Work out the finished part from the listing and answer in its coordinate system (mm). A direction names the side the tool comes from. Coordinates: 2 decimals unless noted, no trailing zeros. Order: outer loops, then holes, each group sorted by start corner. A loop starts at its lowest first (then second) coordinate and runs counter-clockwise, first axis right, second up.
1. Find the intervals of material crossed by probe 1 along Y at (x, z) = (12, -4.75); probe 2 along Y at (x, z) = (9.25, -0.5); probe 3 along Z at (x, y) = (11, -12.75), in increasing order.
2. Flat-ended cylindrical pins translate along their axes: pin 1 Ø7 at (x, y) = (12, -8.5) entering from +Z; pin 2 Ø5 at (x, y) = (6.5, -2.5) entering from +Z; pin 3 Ø1.5 at (y, z) = (-7, -5.5) entering from -X; pin 4 Ø0.7 at (x, z) = (3, -1.5) entering from -Y. Find the tip coordinate at first contact, or state that the pin passes through.
3. The part is cut by section A-A, the plane x = 12.5. Give the vertices of the cut face in (y, z).
4. A tool of negligible diameter and unlimited length cuts with its end or side. For faces 1 (the flat face through (10, 0, -5)), 2 (the flat face through (1, -8, -3.175)), 3 (the flat face through (8, -1.778, -3)), 4 (the flat face through (9.398, -14, -1)), 5 (the flat face through (0, -8, -2)), from which of +Z, -Z, +X, -X, +Y, -Y can it reach the whole face along a straight path? Write none if from no direction.
5. The part is cut by section B-B, the plane y = -8.5. Give the vertices of the cut face in (x, z) (3 decimals), then the cut area to 3 significant figures.
6. The part is cut by section C-C, the plane z = -0.25. Give the vertices of the cut face in (x, y), then the cut area to 3 significant figures.
7. Determine the mould class of faces 6 (the flat face through (8, -13.462, -3)), 7 (the flat face through (10, -15, -2.794)), 8 (the flat face through (10, -1, -2.794)), 9 (the flat face through (4.125, -7.538, -3.091)) for opening direction Z: +Z half, -Z half, draft (parallel to the pull), parting line (faces both ways), or undercut.
```python
from build123d import *

# Parameters (mm, degrees)
BOSS_EXTRUDE1_DEPTH = 15.24
CUT_EXTRUDE1_DEPTH  = 16.748
CUT_EXTRUDE2_DEPTH  = 5.842
FILLET1_R           = 0.762


with BuildPart() as part:
    # Sketch1 → Boss-Extrude1 (new body)
    with BuildSketch(Plane(origin=(0, 0, 0), x_dir=(1, 0, 0), z_dir=(0, 1, 0))):
        Polygon((0, 0), (0, 3.175), (2.413, 3.175), (6.604, 7.366), (15.748, 7.366), (15.748, 2.794), (9.398, 2.794), (9.398, 0), align=None)
    extrude(amount=-BOSS_EXTRUDE1_DEPTH)

    # Sketch5 → Cut-Extrude1 (cut, through all)
    with BuildSketch(Plane.ZY):
        Polygon((0, -1.0033), (0, 0), (-2.794, 0), (-2.794, -1.0033), (-2.2606, -1.0033), (-1.7018, -0.4445), (-1.0922, -0.4445), (-0.5334, -1.0033), align=None)
    cut_extrude1 = extrude(amount=-CUT_EXTRUDE1_DEPTH, mode=Mode.SUBTRACT)

    # Mirror1: Cut-Extrude1 across plane
    add(cut_extrude1.mirror(Plane.ZX.offset(-7.62)), mode=Mode.SUBTRACT)

    # Sketch6 → Cut-Extrude2 (cut, symmetric)
    with BuildSketch(Plane(origin=(0, -7.62, 0), x_dir=(1, 0, 0), z_dir=(0, 1, 0))):
        Polygon((15.748, 6.096), (7.130051224, 6.096), (1.034051224, 0), (15.748, 0), align=None)
    extrude(amount=CUT_EXTRUDE2_DEPTH, both=True, mode=Mode.SUBTRACT)

    # Fillet1
    fillet1_edges = [part.edges().sort_by_distance(p)[0] for p in [
        (11.439025612, -13.462, -6.096),
        (11.439025612, -1.778, -6.096),
        (11.176, -15.24, -7.366),
        (11.176, 0, -7.366),
    ]]
    fillet(fillet1_edges, radius=FILLET1_R)


solid = part.part
```
Geometry says:
1. probe 1: y = -15.24 to -13.46, -1.78 to 0
1. probe 2: y = -14.24 to -13.46, -1.78 to -1
1. probe 3: z = -7.37 to -6.09
2. pin 1: stops at z = -6.1
2. pin 2: stops at z = 0
2. pin 3: stops at x = 3.99
2. pin 4: stops at y = -14.8
3. outline: (-15.24, -6.6) arc R0.76 ccw to (-14.48, -7.37) - (-0.76, -7.37) arc R0.76 ccw to (0, -6.6) - (0, -2.79) - (-1.78, -2.79) - (-1.78, -5.33) arc R0.76 cw to (-2.54, -6.1) - (-12.7, -6.1) arc R0.76 cw to (-13.46, -5.33) - (-13.46, -2.79) - (-15.24, -2.79) - close
4. face 1: +Z, -Z, +X, -X, +Y
4. face 2: -Z, -X, +Y, -Y
4. face 3: +Z, +X
4. face 4: +Z, +X, +Y, -Y
4. face 5: +Z, -Z, -X, +Y, -Y
5. outline: (0, -3.175) - (2.413, -3.175) - (6.604, -7.366) - (15.748, -7.366) - (15.748, -6.096) - (7.13, -6.096) - (1.034, 0) - (0, 0) - close
5. area: 26.0 mm2
6. outline: (0, -14.24) - (9.4, -14.24) - (9.4, -13.46) - (1.28, -13.46) - (1.28, -1.78) - (9.4, -1.78) - (9.4, -1) - (0, -1) - close
6. area: 29.6 mm2
7. face 6: draft
7. face 7: undercut
7. face 8: undercut
7. face 9: +Z half
